```python
from build123d import *

# Parameters (mm, degrees)
CYLINDER093_R     = 1.5
CYLINDER093_DEPTH = 14
CYLINDER090_R     = 11.7
CYLINDER090_DEPTH = 33
CYLINDER094_R     = 1.5
CYLINDER094_DEPTH = 14
CYLINDER088_R     = 14
CYLINDER088_DEPTH = 33
BOX016_W          = 1
BOX016_H          = 1
BOX016_DEPTH      = 1
CYLINDER084_R     = 17
CYLINDER084_DEPTH = 5
CYLINDER095_R     = 11
CYLINDER095_DEPTH = 34
CYLINDER_R        = 18
CYLINDER_DEPTH    = 34


with BuildPart() as obj1:
    # Cylinder093 → Cylinder093 (new body)
    with BuildSketch(Plane(origin=(53.66, 148, -15), x_dir=(1, 0, 0), z_dir=(0, 0, 1))):
        Circle(CYLINDER093_R)
    extrude(amount=CYLINDER093_DEPTH)


with BuildPart() as obj2:
    # Cylinder090 → Cylinder090 (new body)
    with BuildSketch(Plane(origin=(73.66, 148, -10), x_dir=(1, 0, 0), z_dir=(0, 0, 1))):
        Circle(CYLINDER090_R)
    extrude(amount=CYLINDER090_DEPTH)


with BuildPart() as fusion039:
    # Cylinder094 → Cylinder094 (new body)
    with BuildSketch(Plane(origin=(93.66, 148, -14), x_dir=(1, 0, 0), z_dir=(0, 0, 1))):
        Circle(CYLINDER094_R)
    extrude(amount=CYLINDER094_DEPTH)

    # Fusion039: union obj1, obj2
    add(obj1.part)
    add(obj2.part)


with BuildPart() as obj3:
    # Cylinder088 → Cylinder088 (new body)
    with BuildSketch(Plane(origin=(73.66, 148, -10), x_dir=(1, 0, 0), z_dir=(0, 0, 1))):
        Circle(CYLINDER088_R)
    extrude(amount=CYLINDER088_DEPTH)


with BuildPart() as obj4:
    # Box016 → Box016 (new body)
    with BuildSketch(Plane(origin=(63, 136, -8), x_dir=(1, 0, 0), z_dir=(0, 0, 1))):
        with Locations((0.5, 0.5)):
            Rectangle(BOX016_W, BOX016_H)
    extrude(amount=BOX016_DEPTH)


with BuildPart() as obj5:
    # Cylinder084 → Cylinder084 (new body)
    with BuildSketch(Plane(origin=(73.66, 148, -10), x_dir=(1, 0, 0), z_dir=(0, 0, 1))):
        Circle(CYLINDER084_R)
    extrude(amount=CYLINDER084_DEPTH)

    # Fusion038: union obj3, obj4
    add(obj3.part)
    add(obj4.part)

    # Cut010: cut Fusion039
    add(fusion039.part, mode=Mode.SUBTRACT)


with BuildPart() as obj5_1:
    # Cut010 placement: moved
    add(obj5.part.moved(Location((-73.66, -148, -23))))


with BuildPart() as fusion:
    # Cylinder095 → Cylinder095 (new body)
    with BuildSketch(Plane.XY.offset(-33)):
        Circle(CYLINDER095_R)
    extrude(amount=CYLINDER095_DEPTH)

    # Fusion: union obj5
    add(obj5_1.part)


with BuildPart() as cut:
    # Cylinder → Cylinder (new body)
    with BuildSketch(Plane.XY.offset(-33)):
        Circle(CYLINDER_R)
    extrude(amount=CYLINDER_DEPTH)

    # Cut: cut Fusion
    add(fusion.part, mode=Mode.SUBTRACT)


solid = cut.part
```
For this review, take the finished solid that the model builds, in its own axes (mm). A direction names the side the tool comes from. Coordinates: 2 decimals unless noted, no trailing zeros. Order: outer loops, then holes, each group sorted by start corner. A loop starts at its lowest first (then second) coordinate and runs counter-clockwise, first axis right, second up. Notation, with made-up numbers: (-19, 14) -> (4, 14) arc R22 cw to (4, 41) -> close; hole circle Ø10 at (-12.75, 51.25). An arc over 180 degrees is marked (long way). Use CSV: the item, a comma, the result in double quotes. Start each with the question number.
Item 1: For faces 4 (the face through (5.4, -10.38, -16.73)), 5 (the face through (16, -7, -33)), list the 3-axis set-ups (+Z, -Z, +X, -X, +Y, -Y) from which the entire face can be reached by the end or side of a thin tool; tool diameter is ignored.
Item 2: Wall thickness on probe 1 along Y at (x, z) = (0, -15.5); probe 2 along Y at (x, z) = (0, -29.45); probe 3 along X at (y, z) = (2, -10.5): over which ranges is each line inside the solid? List them lowest first.
Item 3: We need section D-D, the plane x = -14.5. Give the boundary of the cut face in (y, z).
Item 4: We need section A-A, the plane z = -5. Give the boundary of the cut face in (x, y), then the cut area to 3 significant figures.
Item 5: Draft analysis for pull direction Y (two halves, no side actions). For faces 1 (the face through (-2.343, 17.847, -16.238)), 2 (the face through (8, -15, -31)), 3 (the face through (-8, -8, 1)), state which applies: pulls with the +Y half, pulls with the -Y half, needs draft (parallel to the pull), parting line crosses it, or undercut.
Item 6: We need section B-B, the plane y = 0. Give the boundary of the cut face in (x, z).
Item 7: Insertion check: pin 1 (12 mm diameter, centred on x = 11, y = -5, fed in from -Z); pin 2 (4 mm diameter, centred on x = -8, y = 1.5, fed in from +Z); pin 3 (1.5 mm diameter, centred on y = -13.5, z = -17, fed in from -X); pin 4 (1.5 mm diameter, centred on x = -9.5, z = -23, fed in from +Y). Each pin has a flat end and moves straight along its axis. Give the tip position at first contact, or say it passes through.
Derived:
1,face 4,"-Z"
1,face 5,"-Z, +X, -X, +Y, -Y"
2,probe 1,"y = -18 to -14, -11.7 to -11, 11 to 11.7, 14 to 18"
2,probe 2,"y = -18 to -17, -11.7 to -11, 11 to 11.7, 17 to 18"
2,probe 3,"x = -17.89 to -13.86, -11.53 to -10.82, 10.82 to 11.53, 13.86 to 17.89"
3,outline,"(-10.67, -33) -> (-8.87, -33) -> (-8.87, -28) -> (8.87, -28) -> (8.87, -33) -> (10.67, -33) -> (10.67, 1) -> (-10.67, 1) -> close"
4,outline,"circle Ø36 at (0, 0); circle Ø23.4 at (0, 0); hole circle Ø28 at (0, 0); hole circle Ø22 at (0, 0)"
4,area,"452 mm^2"
5,face 1,"parting line crosses it"
5,face 2,"undercut"
5,face 3,"needs draft"
6,outline,"(-18, -33) -> (-17, -33) -> (-17, -28) -> (-14, -28) -> (-14, 0) -> (-11.7, 0) -> (-11.7, -33) -> (-11, -33) -> (-11, 1) -> (-18, 1) -> close; (11, -33) -> (11.7, -33) -> (11.7, 0) -> (14, 0) -> (14, -28) -> (17, -28) -> (17, -33) -> (18, -33) -> (18, 1) -> (11, 1) -> close"
7,pin 1,"stops at z = -33"
7,pin 2,"passes through"
7,pin 3,"stops at x = -12.71"
7,pin 4,"stops at y = 15.73"
